Verification items for the finished model (mm, model axes). A direction names the side the tool comes from. Coordinates: 2 decimals unless noted, no trailing zeros. Order: outer loops, then holes, each group sorted by start corner. A loop starts at its lowest first (then second) coordinate and runs counter-clockwise, first axis right, second up. Notation, with made-up numbers: M 30,74 L 56,74 A10 ccw 56,86 Z; hole C 57.5,-5.5 d7. An arc over 180 degrees is marked long. Return JSON: item names as keys, results as strings. Group by question number.
1. Gauge pin test, flat ends, axial feed: pin 1 (8 mm diameter, centred on x = 23.5, z = 1.5, fed in from -Y); pin 2 (10 mm diameter, centred on x = 29, z = 2.5, fed in from -Y); pin 3 (6 mm diameter, centred on x = 26.5, y = 0.5, fed in from -Z). Record the tip position at first contact, or that the pin passes through.
2. Set-up check for faces 4 (the cylindrical face through (0.36, 3.66, -16.59)), 5 (the cylindrical face through (-0.206, -2.517, 0.011)), 6 (the cylindrical face through (3.72, 2.91, 15.78)), 7 (the flat face through (3.18, -3.44, 3.92)): record each of +Z, -Z, +X, -X, +Y, -Y from which the full face is reachable in a straight line by a thin tool's end or side.
3. Mould release check, pull along Y, two halves, no side actions. Record for faces 1 (the flat face through (3.18, -3.44, 15.65)), 2 (the cylindrical face through (3.72, 2.91, -15.78)), 3 (the flat face through (18.175, -0.015, -16.565)): +Y half, -Y half, draft (parallel to the pull), parting line (faces both ways), or undercut.
4. Section check B-B, the plane z = -18.5. Record the cut outline in (x, y) (1 decimal), plus the area to 3 significant figures.
5. Material ranges on line 1 along Y through (x, z) = (0, 0.45) (3 decimals); line 2 along Y through (x, z) = (26, 11); line 3 along X through (y, z) = (1, 8.5), recorded low to high.
```python
from build123d import *

# Parameters (mm, degrees)
SKETCH2_R               = 2.54
BOSS_EXTRUDE1_DEPTH     = 22.225
CUT_EXTRUDE1_DEPTH      = 7.35
CUT_EXTRUDE1_DEPTH_BACK = 7.35
SKETCH7_R               = 0.9525
CUT_EXTRUDE5_DEPTH      = 0.9525
CUT_EXTRUDE6_DEPTH      = 14.2875
SKETCH11_R              = 2.8575
BOSS_EXTRUDE2_DEPTH     = 22.225
CUT_EXTRUDE7_DEPTH      = 6.35


with BuildPart() as part:
    # Sketch2 → Boss-Extrude1 (new body, symmetric)
    with BuildSketch(Plane.XY):
        with BuildLine():
            Line((0.635, 6.318170226), (32.0675, 3.159085113))
            ThreePointArc((32.0675, 3.159085113), (34.925, 0), (32.0675, -3.159085113))
            Line((32.0675, -3.159085113), (0.635, -6.318170226))
            ThreePointArc((0.635, -6.318170226), (-6.35, 0), (0.635, 6.318170226))
        make_face()
        with Locations((-1.908273726, 1.920652886)):
            Circle(SKETCH2_R, mode=Mode.SUBTRACT)
    extrude(amount=BOSS_EXTRUDE1_DEPTH, both=True)

    # Sketch3 → Cut-Extrude1 (cut, two sides)
    with BuildSketch(Plane(origin=(0, 0, 0), x_dir=(1, 0, 0), z_dir=(0, 1, 0))) as cut_extrude1_sk:
        Polygon((-6.35, 22.225), (34.925, 12.7), (34.925, 31.680918885), align=None)
        Polygon((-6.35, -22.225), (34.925, -12.7), (34.925, -37.636863469), align=None)
    extrude(amount=CUT_EXTRUDE1_DEPTH, mode=Mode.SUBTRACT)
    extrude(cut_extrude1_sk.sketch, amount=-CUT_EXTRUDE1_DEPTH_BACK, mode=Mode.SUBTRACT)

    # Sketch7 → Cut-Extrude5 (cut, symmetric)
    with BuildSketch(Plane.XY):
        with Locations((0, -1.5875)):
            Circle(SKETCH7_R)
    extrude(amount=CUT_EXTRUDE5_DEPTH, both=True, mode=Mode.SUBTRACT)

    # Sketch5 → Cut-Extrude6 (cut)
    with BuildSketch(Plane.XY.offset(25.4)):
        with BuildLine():
            Line((3.064489009, -0.895879696), (3.299937252, -6.050333954))
            Line((3.299937252, -6.050333954), (5.210798469, -13.210091767))
            Line((5.210798469, -13.210091767), (-7.623273726, -5.718328917))
            Line((-7.623273726, -5.718328917), (-7.623273726, 1.920652886))
            ThreePointArc((-7.623273726, 1.920652886), (-0.451927961, 7.446979153), (3.064489009, -0.895879696))
        make_face()
    cut_extrude6 = extrude(amount=-CUT_EXTRUDE6_DEPTH, mode=Mode.SUBTRACT)

    # Mirror2: Cut-Extrude6 across plane
    add(cut_extrude6.mirror(Plane.XY), mode=Mode.SUBTRACT)

    # Sketch11 → Boss-Extrude2 (add, symmetric)
    with BuildSketch(Plane.XY):
        with Locations(Location((-1.908273726, 1.920652886, 0), (0, 0, 180))):  # turned: the seam where the file's is
            Circle(SKETCH11_R)
    extrude(amount=BOSS_EXTRUDE2_DEPTH, both=True)

    # Sketch9 → Cut-Extrude7 (cut)
    with BuildSketch(Plane.XY.offset(0.79375)):
        Polygon((-4.939406342, 3.990584542), (3.064489009, -0.895879696), (3.299937252, -6.050333954), (-14.496579657, -7.838951202), align=None)
    cut_extrude7 = extrude(amount=CUT_EXTRUDE7_DEPTH, mode=Mode.SUBTRACT)

    # Mirror1: Cut-Extrude7 across plane
    add(cut_extrude7.mirror(Plane.XY), mode=Mode.SUBTRACT)


solid = part.part
```
Answers follow:
{
 "1": {"pin 1": "y = -4.42", "pin 2": "y = -3.97", "pin 3": "z = -15.34"},
 "2": {"face 4": "-Z", "face 5": "none", "face 6": "+Z", "face 7": "-X, -Y"},
 "3": {"face 1": "-Y half", "face 2": "undercut", "face 3": "draft"},
 "4": {"outline": "C -1.9,1.9 d5.7; M 1.9,6.2 A5.7 cw 3.1,-0.9 L 3.3,-6.1 L 9.8,-5.4 L 9.8,5.4 Z", "area": "100 mm^2"},
 "5": {"line 1": "-6.35 to -2.54, -0.635 to 6.35", "line 2": "-3.77 to 3.77", "line 3": "-6.27 to 34.76"}
}
